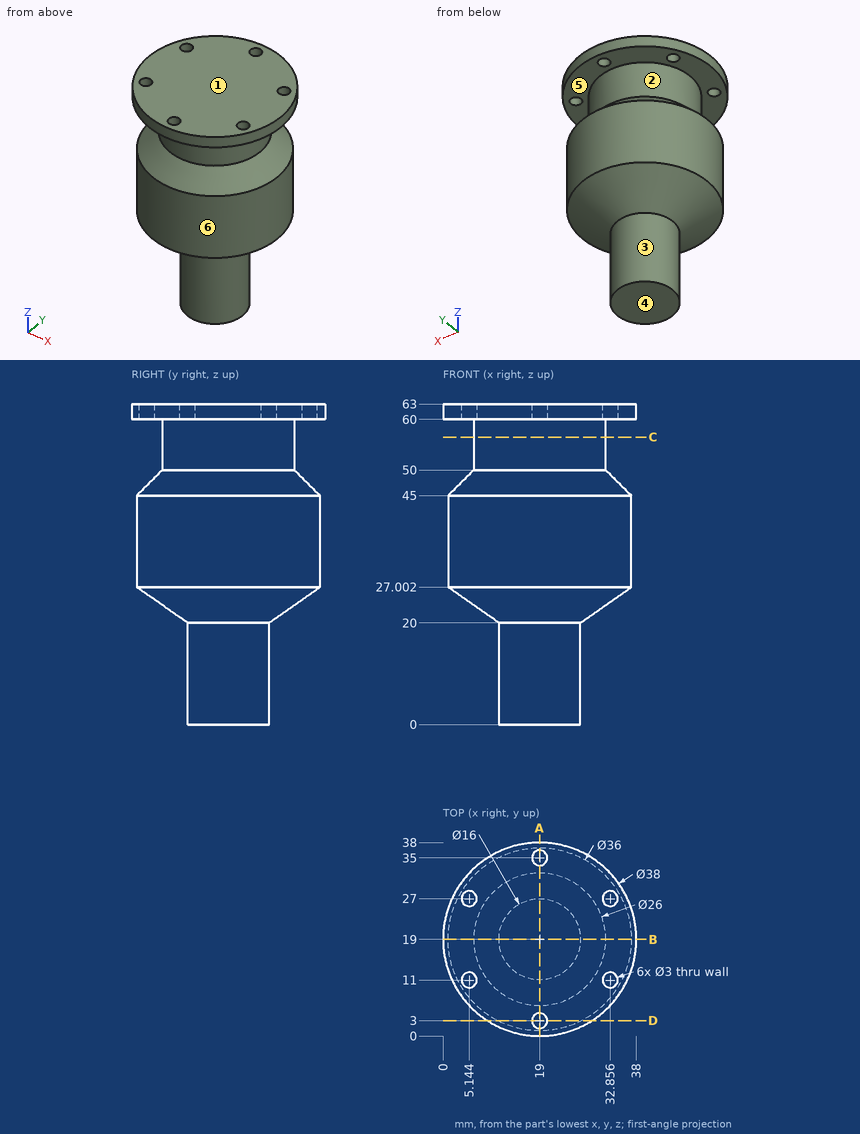
Geometry check sheet. Reference: drawing and pictorial views, mm from the part's lowest x, y, z. A direction names the side the tool comes from. Give positions to 0.01 mm unless a question says otherwise; leave off trailing zeros. Order: outer loops, then holes, each group sorted by start corner. A loop starts at its lowest first (then second) coordinate and runs counter-clockwise, first axis right, second up. Notation, with made-up numbers: M 76.5,49 L 109.5,49 A30 ccw 109.5,84 Z; hole C 74.5,68 d2. An arc over 180 degrees is marked long. Use one line per item in the form item = value. Start each with the question number.
Q1. Go/stop test with flat-tipped pins: pin 1 Ø2 at (x, z) = (34, 42.5) entering from +Y (1 decimal); pin 2 Ø5 at (x, y) = (32.86, 11) entering from -Z; pin 3 Ø2 at (x, y) = (29.5, 6) entering from -Z; pin 4 Ø1.5 at (y, z) = (28, 17) entering from -X. Record where each tip stops, or that it passes through.
Q2. Scan lines: line 1 along Y through (x, z) = (19, 61); line 2 along X through (y, z) = (2, 60.5) (1 decimal); line 3 along Z through (x, y) = (28, 30). Record each from-to range of solid material in increasing order. Write a range as [from, to].
Q3. Access from +Z, -Z, +X, -X, +Y, -Y to the whole of each face (thin tool, end or side, straight path). Record for the marked faces 4, 5 and 6.
Q4. Mould release check, pull along Z, two halves, no side actions. Record for the marked faces 1, 2 and 3: +Z half, -Z half, draft (parallel to the pull), parting line (faces both ways), or undercut.
Q5. Section check A-A (x = 19). Enter the section's corners in (y, z), then the cut area to 3 significant figures.
Q6. Section check D-D (y = 3). Count the separate pieces of the cut face and the enclosed holes in it, then the cut area to 3 significant figures.
Q7. Section check B-B (y = 19). Enter the section's corners in (x, z).
Q8. Section check C-C (z = 56.5). Enter the section's corners in (x, y).
Evaluation:
q1.pin_1 = 30.3
q1.pin_2 = 23.85
q1.pin_3 = 25.4
q1.pin_4 = through
q2.line_1 = [0, 1.5], [4.5, 33.5], [36.5, 38]
q2.line_2 = [10.5, 17.9], [20.1, 27.5]
q2.line_3 = [24.35, 48.79], [60, 63]
q3.face_4 = -Z, +X, -X, +Y, -Y
q3.face_5 = none
q3.face_6 = -Z
q4.face_1 = +Z half
q4.face_2 = undercut
q4.face_3 = draft
q5.outline = M 0,60 L 1.5,60 L 1.5,63 L 0,63 Z; M 1,27 L 11,20 L 11,0 L 27,0 L 27,20 L 37,27 L 37,45 L 32,50 L 32,60 L 33.5,60 L 33.5,63 L 4.5,63 L 4.5,60 L 6,60 L 6,50 L 1,45 Z; M 36.5,60 L 38,60 L 38,63 L 36.5,63 Z
q5.area = 1,660 mm2
q6.separate_pieces = 3
q6.enclosed_holes = 0
q6.area = 386 mm2
q7.outline = M 0,60 L 6,60 L 6,50 L 1,45 L 1,27 L 11,20 L 11,0 L 27,0 L 27,20 L 37,27 L 37,45 L 32,50 L 32,60 L 38,60 L 38,63 L 0,63 Z
q8.outline = C 19,19 d26
